```python
from build123d import *

# Parameters (mm, degrees)
F3_DEPTH = 8
F4_W     = 12.8698311746
F4_H     = 13.9981461689
F5_DEPTH = 3
F6_DEPTH = 3


with BuildPart() as f1:
    # F0 (on Front) → F1 (revolve)
    with BuildSketch(Plane.XZ):
        Polygon((30, 3), (0, 3), (-30, 3), (-30, 0), (0, 0), (30, 0), align=None)
    revolve(axis=Axis((15, 0, 0), (1, 0, 0)))

    # F2 (on face) → F3 (cut)
    with BuildSketch(Plane(origin=(-30, 0, 0), x_dir=(0, -1, 0), z_dir=(-1, 0, 0))):
        with BuildLine():
            Line((3.0024852457, -0.5085919919), (-3.0024852457, -0.5085919919))
            ThreePointArc((-3.0024852457, -0.5085919919), (0, -3.0452558948), (3.0024852457, -0.5085919919))
        make_face()
        with BuildLine():
            ThreePointArc((2.9974451145, 0.5375), (0, 3.0452558948), (-2.9974451145, 0.5375))
            Line((-2.9974451145, 0.5375), (2.9974451145, 0.5375))
        make_face()
    extrude(amount=-F3_DEPTH, mode=Mode.SUBTRACT)

    # F4 (on Top) → F5 (join)
    with BuildSketch(Plane.XY):
        Polygon((29.9149005125, 8), (29.9149005125, 0), (29.9149005125, -8), (44.9149005125, -8), (44.9149005125, 8), align=None)
        with Locations((37.3716000468, 0.0690473244)):
            Rectangle(F4_W, F4_H, mode=Mode.SUBTRACT)
        with Locations((37.3716000468, 0.0690473244)):
            Rectangle(F4_W, F4_H)
    extrude(amount=-F5_DEPTH)

    # F4 (on Top) → F6 (join)
    with BuildSketch(Plane.XY):
        Polygon((29.9149005125, 8), (29.9149005125, 0), (29.9149005125, -8), (44.9149005125, -8), (44.9149005125, 8), align=None)
        with Locations((37.3716000468, 0.0690473244)):
            Rectangle(F4_W, F4_H, mode=Mode.SUBTRACT)
    extrude(amount=F6_DEPTH)


solid = f1.part
```
Input: part model. Units: mm. Frame: model coordinates. A direction names the side the tool comes from. Coordinates: 2 decimals unless noted, no trailing zeros. Write each loop counter-clockwise with the first axis right and the second up, starting at its lowest first coordinate (ties: lowest second). Pieces come first, ordered by that corner, then holes. Notation, with made-up numbers: (20.25, 14.25) - (58.25, 14.25) arc R10 ccw to (58.25, 20.25) - close; hole circle Ø3 at (-3.5, 66.25). An arc over 180 degrees is marked (long way). Put each result on its own line as item: value. Start each with the question number.
1) Reachability of faces 1 (the face through (-26, 0, 0.538)), 2 (the face through (-22, 0, -1)), 3 (the face through (37, 0, -3)), 4 (the face through (37, -6.93, 1)), 5 (the face through (38, 8, 0)) from +Z, -Z, +X, -X, +Y, -Y: full face, straight path, thin tool, end or side. Return the list, or none.
2) Mould query, pull axis Y, two halves, no side actions, for faces 6 (the face through (37, 0, 0)), 7 (the face through (30.6, 0.1, 3)), 8 (the face through (37, -8, 0)), 9 (the face through (0, -3, 0)). Classes: pulls with the +Y half, pulls with the -Y half, needs draft (parallel to the pull), parting line crosses it, or undercut.
3) Cut plane A-A (z = 1.8). Return the cut outline in (x, y).
4) Contact query for flat-ended pins moving along their axis: pin 1 (6.5 mm diameter, centred on x = -26.5, y = -1.5, fed in from -Z); pin 2 (4 mm diameter, centred on x = 2, y = -3.5, fed in from -Z); pin 3 (2 mm diameter, centred on x = -13, z = 2, fed in from -Y). Output: stop coordinate, or through.
5) Cut plane D-D (x = -13.5). Return the cut outline in (y, z), plus the area to 3 significant figures.
6) Cut plane B-B (z = -1.85). Return the cut outline in (x, y), plus the area to 3 significant figures.
7) Ray query, L1, parallel to X at y = 0.5, z = 0.3; L2, parallel to X at y = -5.5, z = 1.25; L3, parallel to X at y = 3, z = -1.15. Return the intervals inside material, ascending.
8) Cut plane C-C (y = -1.25). Return the cut outline in (x, z), plus the area to 3 significant figures.
Resolved:
1. face 1: +Z, -X, +Y, -Y
1. face 2: -Z, -X, +Y, -Y
1. face 3: -Z, +X, -X, +Y, -Y
1. face 4: +Z
1. face 5: +Z, -Z, +X, -X, +Y
2. face 6: undercut
2. face 7: needs draft
2. face 8: pulls with the -Y half
2. face 9: parting line crosses it
3. outline: (-22, -2.4) - (29.91, -2.4) - (29.91, -8) - (44.91, -8) - (44.91, 8) - (29.91, 8) - (29.91, 2.4) - (-22, 2.4) - close; hole (30.94, -6.93) - (43.81, -6.93) - (43.81, 7.07) - (30.94, 7.07) - close
4. pin 1: stops at z = -0.51
4. pin 2: stops at z = -2.6
4. pin 3: stops at y = -2.83
5. outline: circle Ø6 at (0, 0)
5. area: 28.3 mm2
6. outline: (-22, -2.36) - (29.91, -2.36) - (29.91, -8) - (44.91, -8) - (44.91, 8) - (29.91, 8) - (29.91, 2.36) - (-22, 2.36) - close
6. area: 485 mm2
7. L1: x = -30 to 30.94, 43.81 to 44.91
7. L2: x = 29.91 to 30.94, 43.81 to 44.91
7. L3: x = 29.91 to 44.91
8. outline: (-30, -0.51) - (-22, -0.51) - (-22, -2.73) - (29.91, -2.73) - (29.91, -3) - (44.91, -3) - (44.91, 3) - (43.81, 3) - (43.81, 0) - (30.94, 0) - (30.94, 3) - (29.91, 3) - (29.91, 2.73) - (-22, 2.73) - (-22, 0.54) - (-30, 0.54) - close
8. area: 343 mm2
